from build123d import *

# Parameters (mm, degrees)
F0_R     = 7.9
F0_R_2   = 6.35
F1_DEPTH = 15.875
F0_R_3   = 2.8575
F2_DEPTH = 46.228
F0_R_4   = 16.1925
F0_R_5   = 1.905
F4_DEPTH = 3.175
F6_DEPTH = 2.2


with BuildPart() as f1:
    # F0 (on Top) → F1 (new body)
    with BuildSketch(Plane.XY):
        Circle(F0_R)
        Circle(F0_R_2, mode=Mode.SUBTRACT)
    extrude(amount=F1_DEPTH)

    # F0 (on Top) → F2 (join)
    with BuildSketch(Plane.XY):
        Circle(F0_R_2)
        Circle(F0_R_3, mode=Mode.SUBTRACT)
    extrude(amount=F2_DEPTH)

    # F0 (on Top) → F4 (join)
    with BuildSketch(Plane.XY):
        Circle(F0_R_4)
        with Locations((0, -11.7475)):
            Circle(F0_R_5, mode=Mode.SUBTRACT)
        with Locations((-11.7475, 0)):
            Circle(F0_R_5, mode=Mode.SUBTRACT)
        Circle(F0_R, mode=Mode.SUBTRACT)
        with Locations((11.7475, 0)):
            Circle(F0_R_5, mode=Mode.SUBTRACT)
        with Locations((0, 11.7475)):
            Circle(F0_R_5, mode=Mode.SUBTRACT)
    extrude(amount=F4_DEPTH)

    # F5 (on face) → F6 (cut)
    with BuildSketch(Plane.XY.offset(46.228)):
        with BuildLine():
            ThreePointArc((6.35, 0), (6.3259541524, 0.5520906279), (6.2539987208, 1.1))
            Line((6.2539987208, 1.1), (2.637291461, 1.1))
            ThreePointArc((2.637291461, 1.1), (2.8019070827, 0.5609126048), (2.8575, 0))
            ThreePointArc((2.8575, 0), (2.8019070827, -0.5609126048), (2.637291461, -1.1))
            Line((2.637291461, -1.1), (6.2539987208, -1.1))
            ThreePointArc((6.2539987208, -1.1), (6.3259541524, -0.5520906279), (6.35, 0))
        make_face()
        with BuildLine():
            Line((-2.637291461, 1.1), (-6.2539987208, 1.1))
            ThreePointArc((-6.2539987208, 1.1), (-6.35, 0), (-6.2539987208, -1.1))
            Line((-6.2539987208, -1.1), (-2.637291461, -1.1))
            ThreePointArc((-2.637291461, -1.1), (-2.8575, 0), (-2.637291461, 1.1))
        make_face()
    extrude(amount=-F6_DEPTH, mode=Mode.SUBTRACT)


solid = f1.part
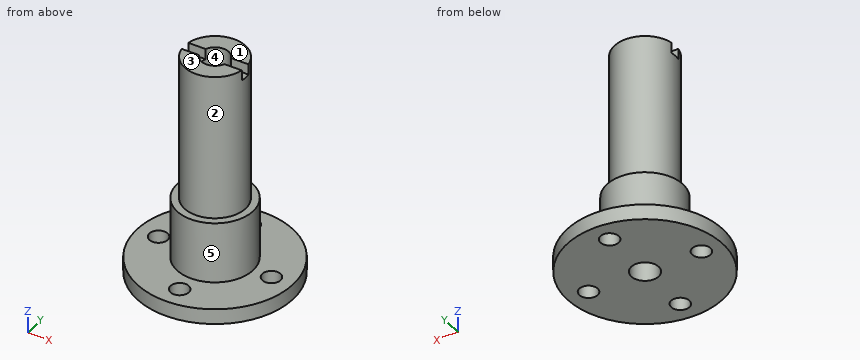
Geometry: final body of the model. Coordinates: model frame, mm. Face numbers are marked on the shaded views. A direction names the side the tool comes from. Coordinates: 2 decimals unless noted, no trailing zeros. Order: outer loops, then holes, each group sorted by start corner. A loop starts at its lowest first (then second) coordinate and runs counter-clockwise, first axis right, second up. Notation, with made-up numbers: M 59.25,-3.75 L 74.25,-3.75 A13 cw 74.25,2.25 Z; hole C 35.5,-33 d8. An arc over 180 degrees is marked long. One line per question, with ' | ' between items. Start each with the question number.
Item 1: Draft query along Y for the marked faces 3, 4 and 5. Return one class per face: released by +Y, released by -Y, zero draft, split by the parting line, or undercut.
Item 2: Pin query (flat end, axial travel): pin 1 Ø1 at (x, y) = (-10.5, 3) entering from +Z (3 decimals); pin 2 Ø2.5 at (x, z) = (-5, 45) entering from +Y; pin 3 Ø1.1 at (x, y) = (4.5, 0) entering from +Z; pin 4 Ø12 at (x, y) = (3.5, 11.5) entering from -Z. Return the tip coordinate at first contact, or that it passes through.
Item 3: Set-up query: the marked faces 1 and 2. Return all of +Z, -Z, +X, -X, +Y, -Y with unobstructed straight access to the full face (end or side cutting, diameter ignored); none if empty.
Item 4: Cut plane A-A, the plane x = 0. Count the separate pieces of the cut face and the enclosed holes in it, then the cut area to 3 significant figures.
Item 5: Ray query, probe 1 along X at (y, z) = (0, 20); probe 2 along Z at (x, y) = (-12, 3) (3 decimals); probe 3 along Z at (x, y) = (2.5, 6.5) (3 decimals). Return the intervals inside material, ascending. Write a range as [from, to].
Item 6: Cut plane C-C, the plane x = 4. Return the cut outline in (y, z) (3 decimals), then the cut area to 3 significant figures.
Item 7: Cut plane D-D, the plane z = 5. Return the cut outline in (x, y) (1 decimal).
A:
1) face 3: zero draft | face 4: undercut | face 5: split by the parting line
2) pin 1: stops at z = 3.175 | pin 2: stops at y = 5.12 | pin 3: stops at z = 44.03 | pin 4: stops at z = 0
3) face 1: +Z, +X, -X, +Y, -Y | face 2: +Z
4) separate pieces: 4 | enclosed holes: 0 | area: 401 mm2
5) probe 1: x = [-6.35, -2.86], [2.86, 6.35] | probe 2: z = [0, 3.175] | probe 3: z = [0, 15.875]
6) outline: M -15.691,0 L 15.691,0 L 15.691,3.175 L 6.812,3.175 L 6.812,15.875 L 4.932,15.875 L 4.932,46.228 L 1.1,46.228 L 1.1,44.028 L -1.1,44.028 L -1.1,46.228 L -4.932,46.228 L -4.932,15.875 L -6.812,15.875 L -6.812,3.175 L -15.691,3.175 Z | area: 567 mm2
7) outline: C 0,0 d15.8; hole C 0,0 d5.7
